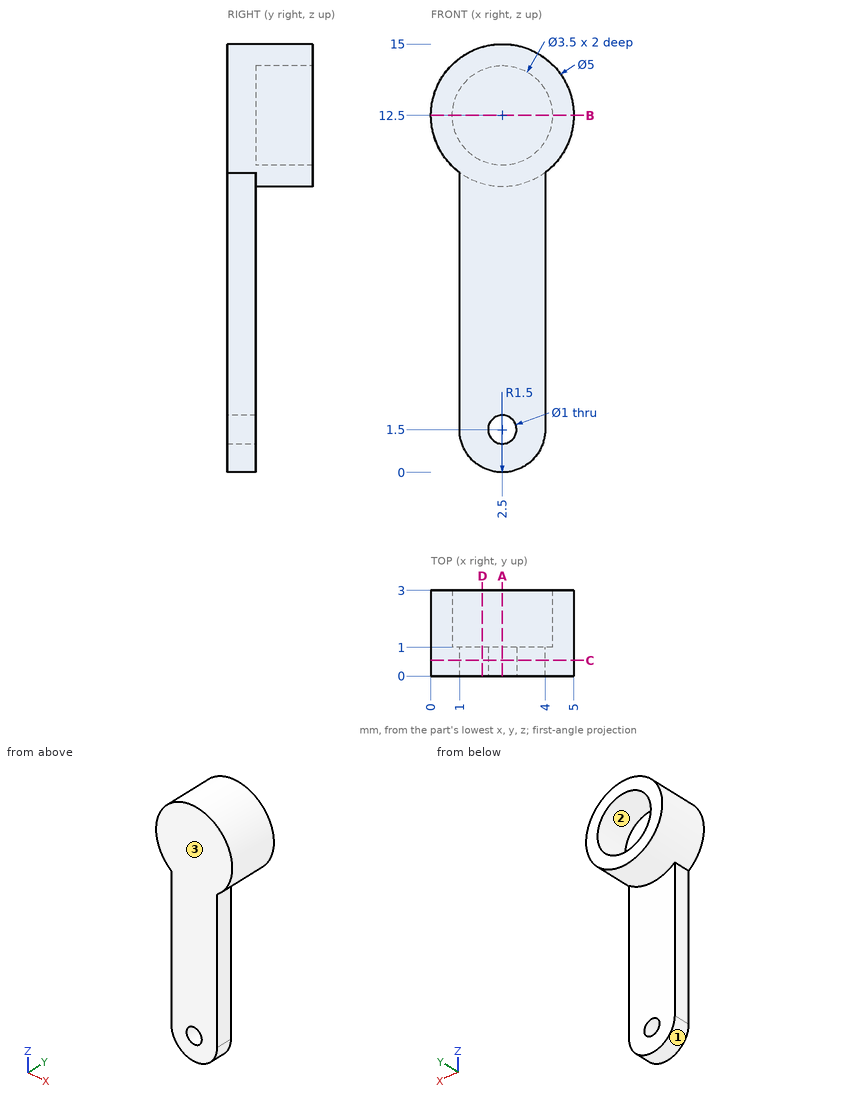
Design review of the part shown in the three views and the two pictorial views. Dimensions are in mm from the part's minimum x, y and z. Round coordinates to 2 decimals unless told otherwise and drop trailing zeros. Loops run counter-clockwise (first coordinate to the right, second up) from the corner with the lowest first, then second, coordinate; pieces in that order, holes last. Notation, with made-up numbers: (-19.75, 12) - (-15.75, 12) arc R25 ccw to (-15.75, 36) - close; hole circle Ø10 at (20.25, 87). An arc over 180 degrees is marked (long way). Answer as CSV lines item,"result".
(1) Mouldability with a two-part tool opening along X and no side actions: class the marked faces 1, 2 and 3 as +X half, -X half, draft (parallel to the pull), parting line (faces both ways), or undercut.
Checked values:
face 1,"parting line"
face 2,"undercut"
face 3,"draft"
(2) Consider section A-A on x = 2.5. Give the boundary of the cut face in (y, z).
Checked values:
outline,"(0, 0) - (1, 0) - (1, 1) - (0, 1) - close; (0, 2) - (1, 2) - (1, 10) - (3, 10) - (3, 10.75) - (1, 10.75) - (1, 14.25) - (3, 14.25) - (3, 15) - (0, 15) - close"
(3) Wall thickness on line 1 (X direction, y = 0.85, z = 1.5); line 2 (X direction, y = 2, z = 12.5); line 3 (X direction, y = 0.6, z = 8): over which ranges is each line inside the solid? List them lowest first.
Checked values:
line 1,"x = 1 to 2, 3 to 4"
line 2,"x = 0 to 0.75, 4.25 to 5"
line 3,"x = 1 to 4"
(4) Consider section B-B on z = 12.5. Give the boundary of the cut face in (x, y), then the cut area to 3 significant figures.
Checked values:
outline,"(0, 0) - (5, 0) - (5, 3) - (4.25, 3) - (4.25, 1) - (0.75, 1) - (0.75, 3) - (0, 3) - close"
area,"8.00 mm2"
(5) Consider section D-D on x = 1.8. Give the boundary of the cut face in (y, z), then the cut area to 3 significant figures.
Checked values:
outline,"(0, 0.17) - (1, 0.17) - (1, 10.1) - (3, 10.1) - (3, 10.9) - (1, 10.9) - (1, 14.1) - (3, 14.1) - (3, 14.9) - (0, 14.9) - close"
area,"17.9 mm2"
(6) Consider section C-C on y = 0.55. Give the boundary of the cut face in (x, z), then the cut area to 3 significant figures.
Checked values:
outline,"(1, 1.5) arc R1.5 ccw to (4, 1.5) - (4, 10.5) arc R2.5 ccw (long way) to (1, 10.5) - close; hole circle Ø1 at (2.5, 1.5)"
area,"48.4 mm2"
(7) Insertion check: P1, Ø1.5, axis at y = 1.5, z = 5.5, coming from the -X side; P2, Ø1.5, axis at x = 2.5, z = 9, coming from the +Y side. Each pin has a flat end and moves straight along its axis. Give the tip position at first contact, or say it passes through.
Checked values:
P1,"stops at x = 1"
P2,"stops at y = 1"
